Geometry: final body of the model. Coordinates: model frame, mm. A direction names the side the tool comes from. Round coordinates to 2 decimals unless told otherwise and drop trailing zeros. Write each loop counter-clockwise with the first axis right and the second up, starting at its lowest first coordinate (ties: lowest second). Pieces come first, ordered by that corner, then holes.
from build123d import *

# Parameters (mm, degrees)
F0_W     = 58.4211573005
F0_H     = 44.2717149854
F1_DEPTH = 25.4
F1_TAPER = -15
F2_DEPTH = 46.482
F4_DEPTH = 25.4


with BuildPart() as f1:
    # F0 (on Front) → F1 (new body)
    with BuildSketch(Plane.XZ):
        with Locations((29.2105786502, 22.1358574927)):
            Rectangle(F0_W, F0_H)
    extrude(amount=F1_DEPTH, taper=F1_TAPER)

    # F2 (add): a face of the model
    f2_faces = [f1.faces().sort_by_distance(p)[0] for p in [
        (29.2105786502, -25.4, 22.1358574927),
    ]]
    extrude(f2_faces, amount=F2_DEPTH)

    # F3 (on face) → F4 (join)
    with BuildSketch(Plane.XZ.offset(71.882)):
        Polygon((18.6991244555, 36.0079780221), (20.2949475497, 25.0953584909), (36.1699461937, 25.0953584909), (36.1699461937, 36.0079780221), align=None)
    extrude(amount=F4_DEPTH)


solid = f1.part
1) Section A-A on y = -87.5. Output: boundary loops of the cut face in (x, z), plus the area to 3 significant figures.
2) First-contact query: P1, Ø1.5, axis at x = 25, y = -20, coming from the +Z side; P2, Ø12, axis at y = -85.5, z = 29, coming from the +X side; P3, Ø1, axis at x = 32.5, z = 15, coming from the -Y side. Flat tips, straight axial feed; report the tip coordinate or a pass-through.
3) Line query: probe 1 along Y at (x, z) = (3.5, 19.5); probe 2 along X at (y, z) = (-6.5, 36.5); probe 3 along Z at (x, y) = (47, -21.5). Output: solid intervals per line, ascending.
4) Reachability of faces 1 (the flat face through (19.486, -84.404, 30.628)), 2 (the flat face through (36.17, -84, 30)), 3 (the flat face through (28, -84, 25.095)) from +Z, -Z, +X, -X, +Y, -Y: full face, straight path, thin tool, end or side. Return the list, or none.
Filled in:
1. outline: (18.7, 36.01) - (20.29, 25.1) - (36.17, 25.1) - (36.17, 36.01) - close
1. area: 182 mm2
2. P1: stops at z = 49.83
2. P2: stops at x = 36.17
2. P3: stops at y = -71.88
3. probe 1: y = -71.88 to 0
3. probe 2: x = -1.74 to 60.16
3. probe 3: z = -5.76 to 50.03
4. face 1: -Z, -X, -Y
4. face 2: +Z, -Z, +X, -Y
4. face 3: -Z, +X, -X, -Y
